Can you work these out from the model? Positions are in its coordinate system, mm. Give positions to 0.01 mm unless a question says otherwise; leave off trailing zeros. Loops run counter-clockwise (first coordinate to the right, second up) from the corner with the lowest first, then second, coordinate; pieces in that order, holes last. Notation, with made-up numbers: (83.5, -33) - (92.5, -33) arc R9 ccw to (92.5, -18) - close; hole circle Ø2 at (-0.75, 77.25). An arc over 180 degrees is marked (long way). Write item = value, one per line.
from build123d import *

# Parameters (mm, degrees)
SKETCH1_W               = 66.5
SKETCH1_H               = 27
BOSS_EXTRUDE1_DEPTH     = 1
CUT_EXTRUDE1_DEPTH      = 72.779175253
CUT_EXTRUDE1_DEPTH_BACK = 10
SKETCH2_W               = 6.707780704
SKETCH2_H               = 1
SKETCH3_R               = 2
CUT_EXTRUDE2_DEPTH      = 72.779175253


with BuildPart() as part:
    # Sketch1 → Boss-Extrude1 (new body)
    with BuildSketch(Plane(origin=(0, 0, 0), x_dir=(1, 0, 0), z_dir=(0, 1, 0))):
        with Locations((33.25, 13.5)):
            Rectangle(SKETCH1_W, SKETCH1_H)
    extrude(amount=BOSS_EXTRUDE1_DEPTH)

    # Sketch2 → Cut-Extrude1 (cut, two sides: drawn at the far end of the back side and taken through both)
    with BuildSketch(Plane(origin=(66.5, 0, 0), x_dir=(0, 0, -1), z_dir=(1, 0, 0)).offset(-CUT_EXTRUDE1_DEPTH_BACK)):
        with Locations((13.5, 0.5)):
            Rectangle(SKETCH2_W, SKETCH2_H)
    extrude(amount=CUT_EXTRUDE1_DEPTH + CUT_EXTRUDE1_DEPTH_BACK, mode=Mode.SUBTRACT)

    # Sketch3 → Cut-Extrude2 (cut, through all)
    with BuildSketch(Plane(origin=(0, 1, 0), x_dir=(1, 0, 0), z_dir=(0, 1, 0))):
        with Locations(Location((63.591245105, 4.5, 0), (0, 0, 270))):
            Circle(SKETCH3_R)
        with Locations(Location((63.591245105, 22.5, 0), (0, 0, 270))):
            Circle(SKETCH3_R)
        with Locations(Location((3.812777096, 22.5, 0), (0, 0, 270))):
            Circle(SKETCH3_R)
        with Locations(Location((3.812777096, 4.5, 0), (0, 0, 270))):
            Circle(SKETCH3_R)
    extrude(amount=-CUT_EXTRUDE2_DEPTH, mode=Mode.SUBTRACT)


solid = part.part
Q1. Imagine slicing it at A-A, the plane z = -22.5. Write out the boundary of the cut face in (x, y), then the cut area to 3 significant figures.
Output:
outline = (0, 0) - (1.81, 0) - (1.81, 1) - (0, 1) - close; (5.81, 0) - (61.59, 0) - (61.59, 1) - (5.81, 1) - close; (65.59, 0) - (66.5, 0) - (66.5, 1) - (65.59, 1) - close
area = 58.5 mm2
Q2. We'd pull the mould along X, two halves only. Please class faces 1 (the cylindrical face through (2.6, 0.51, -6.09)), 2 (the flat face through (33, 1, -14)): released by +X, released by -X, zero draft, split by the parting line, or undercut.
Output:
face_1 = undercut
face_2 = zero draft
Q3. For pin 1 (3.5 mm diameter, centred on x = 3.81, z = -4.5, fed in from +Y), with a flat end and sliding along its axis, tell me the tip position at first contact or that it passes through.
Output:
pin_1 = through
Q4. I need wall thicknesses on L1, parallel to X at y = 0.6, z = -22.5; L2, parallel to X at y = 0.7, z = -23.5; L3, parallel to Z at x = 58, y = 0.3. Which ranges of each line are inside material? Lowest first, please.
Output:
L1 = 0 to 1.81, 5.81 to 61.59, 65.59 to 66.5
L2 = 0 to 2.08, 5.54 to 61.86, 65.32 to 66.5
L3 = -27 to -16.85, -10.15 to 0
Q5. Imagine slicing it at B-B, the plane y = 0.2. Write out the boundary of the cut face in (x, z).
Output:
outline = (0, -27) - (66.5, -27) - (66.5, -16.85) - (56.5, -16.85) - (56.5, -10.15) - (66.5, -10.15) - (66.5, 0) - (0, 0) - close; hole circle Ø4 at (3.81, -22.5); hole circle Ø4 at (3.81, -4.5); hole circle Ø4 at (63.59, -22.5); hole circle Ø4 at (63.59, -4.5)
Q6. Imagine slicing it at C-C, the plane z = -16.25. Write out the boundary of the cut face in (x, y).
Output:
outline = (0, 0) - (56.5, 0) - (56.5, 1) - (0, 1) - close
Q7. Imagine slicing it at D-D, the plane z = -5.5. Write out the boundary of the cut face in (x, y), then the cut area to 3 significant figures.
Output:
outline = (0, 0) - (2.08, 0) - (2.08, 1) - (0, 1) - close; (5.54, 0) - (61.86, 0) - (61.86, 1) - (5.54, 1) - close; (65.32, 0) - (66.5, 0) - (66.5, 1) - (65.32, 1) - close
area = 59.6 mm2
